Geometry: final body of the model. Coordinates: model frame, mm. Face numbers are marked on the shaded views. A direction names the side the tool comes from. Coordinates: 2 decimals unless noted, no trailing zeros. Order: outer loops, then holes, each group sorted by start corner. A loop starts at its lowest first (then second) coordinate and runs counter-clockwise, first axis right, second up. Notation, with made-up numbers: M 30.5,-17 L 38.5,-17 A23 ccw 38.5,15 Z; hole C 61,-8.75 d10. An arc over 180 degrees is marked long. Use CSV: the item, a comma, the result in double quotes. Start each with the question number.
Q1. Access query for the marked faces 1, 2 and 3. Directions: +Z, -Z, +X, -X, +Y, -Y. A direction counts if a zero-diameter tool reaches every point of the face in a straight line with its end or side. Return the directions, or none.
Q2. Section query C-C, the plane x = 45. Output: boundary loops of the cut face in (y, z).
Q3. Section query D-D, the plane z = 32.5. Output: boundary loops of the cut face in (x, y) (3 decimals), and give its area (3 significant figures).
Q4. First-contact query: P1, Ø14.5, axis at x = 19.5, y = -35, coming from the +Z side (3 decimals); P2, Ø10.5, axis at x = 44, y = -21, coming from the +Z side; P3, Ø1.5, axis at x = 8.5, z = 34, coming from the +Y side. Flat tips, straight axial feed; report the tip coordinate or a pass-through.
Q5. Section query A-A, the plane z = 22.5. Output: boundary loops of the cut face in (x, y) (3 decimals), and give its area (3 significant figures).
Q6. Ray query, probe 1 along X at (y, z) = (-62.5, 18) (3 decimals); probe 2 along Z at (x, y) = (4, -31.5); probe 3 along Z at (x, y) = (25.5, -71) (3 decimals). Return the intervals inside material, ascending.
Q7. Section query B-B, the plane y = -21. Output: boundary loops of the cut face in (x, z) (3 decimals), and give its area (3 significant figures).
from build123d import *

# Parameters (mm, degrees)
F0_W     = 77.7748
F0_H     = 9.525
F1_DEPTH = 23.8125
F2_DEPTH = 9.525


with BuildPart() as f1:
    # F0 (on Right) → F1 (new body)
    with BuildSketch(Plane.YZ):
        with Locations((-38.8874, 4.7625)):
            Rectangle(F0_W, F0_H)
    extrude(amount=F1_DEPTH)

    # F0 (on Right) → F2 (join)
    with BuildSketch(Plane.YZ):
        with Locations((-38.8874, 4.7625)):
            Rectangle(F0_W, F0_H)
        Polygon((-77.7748, 38.1), (-77.7748, 9.525), (0, 9.525), (0, 19.05), (-42.8498, 19.05), (-58.7248, 38.1), align=None)
    extrude(amount=F2_DEPTH)

    # F3: F1 across face


with BuildPart() as f1_1:
    add(f1.part)
    add(f1.part.mirror(Plane(origin=(23.8125, -38.8874, 4.7625), x_dir=(0, 1, 0), z_dir=(1, 0, 0))))


solid = f1_1.part
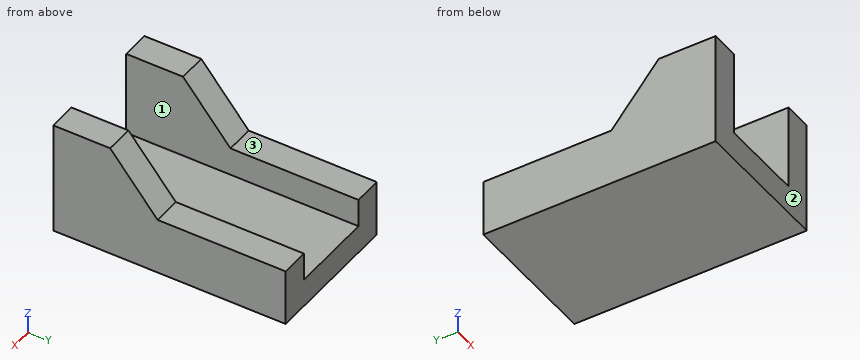
Responses:
1,face 1,"+Z, +Y, -Y"
1,face 2,"+Z, -Z, +X, -X, -Y"
1,face 3,"+Z, +X, -X, +Y"
2,outline,"M -77.77,0 L 0,0 L 0,19.05 L -42.85,19.05 L -58.72,38.1 L -77.77,38.1 Z"
3,outline,"M 0,-77.775 L 9.525,-77.775 L 9.525,-54.058 L 0,-54.058 Z; M 38.1,-77.775 L 47.625,-77.775 L 47.625,-54.058 L 38.1,-54.058 Z"
3,area,"452 mm²"
4,P1,"stops at z = 9.525"
4,P2,"stops at z = 19.05"
4,P3,"stops at y = -54.68"
5,outline,"M 0,-77.775 L 9.525,-77.775 L 9.525,-45.725 L 0,-45.725 Z; M 38.1,-77.775 L 47.625,-77.775 L 47.625,-45.725 L 38.1,-45.725 Z"
5,area,"611 mm²"
6,probe 1,"x = 0 to 9.525, 38.1 to 47.625"
6,probe 2,"z = 0 to 19.05"
6,probe 3,"z = 0 to 9.525"
7,outline,"M 0,0 L 47.625,0 L 47.625,19.05 L 38.1,19.05 L 38.1,9.525 L 9.525,9.525 L 9.525,19.05 L 0,19.05 Z"
7,area,"635 mm²"
